Input: dimensioned drawing with shaded views. Units: mm. Origin: part minimum x, y, z. A direction names the side the tool comes from. Round coordinates to 2 decimals unless told otherwise and drop trailing zeros. Loops run counter-clockwise (first coordinate to the right, second up) from the corner with the lowest first, then second, coordinate; pieces in that order, holes last. Notation, with made-up numbers: (58.5, 38) -> (89.5, 38) arc R23 cw to (89.5, 76) -> close; hole circle Ø8 at (60, 79.25). An arc over 180 degrees is marked (long way). Answer as a JSON object with one key per item and string values.
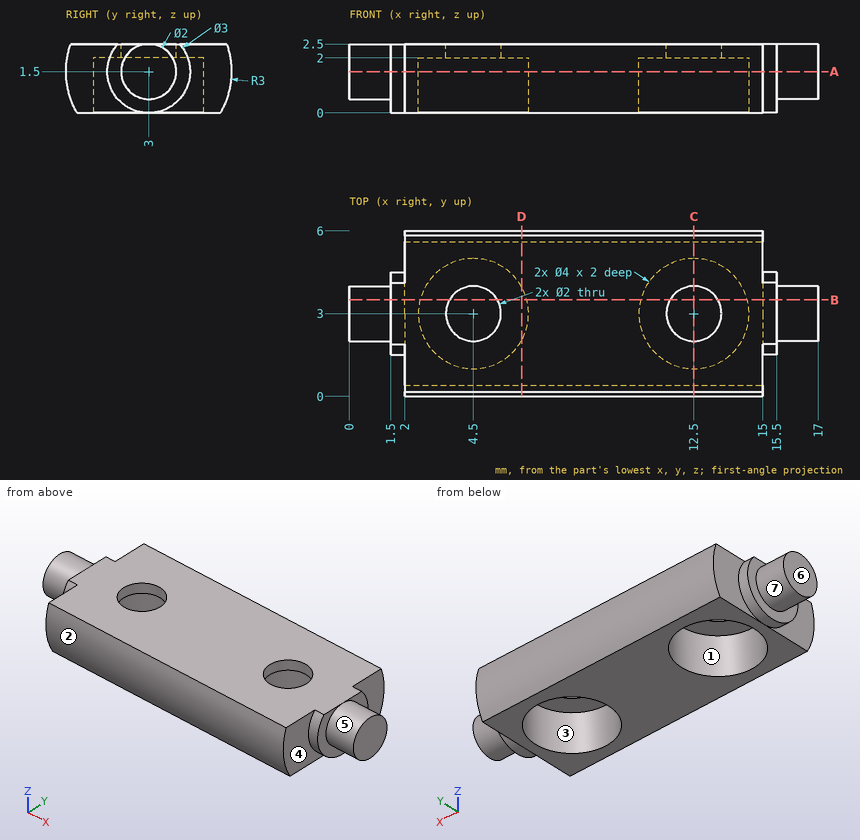
1) Reachability of the marked faces 5, 6 and 7 from +Z, -Z, +X, -X, +Y, -Y: full face, straight path, thin tool, end or side. Return the list, or none.
Output:
{"face 5": "+X", "face 6": "+Z, -Z, -X, +Y, -Y", "face 7": "-X"}
2) Section B-B, the plane y = 3.5. Count the separate pieces of the cut face and the enclosed holes in it, plus the area to 3 significant figures.
Output:
{"separate pieces": "3", "enclosed holes": "0", "area": "22.9 mm^2"}
3) Ray query, probe 1 along X at (y, z) = (3, 0.8); probe 2 along X at (y, z) = (1.5, 0.35); probe 3 along Y at (x, z) = (12.5, 1.4). Return the intervals inside material, ascending.
Output:
{"probe 1": "x = 0 to 2.5, 6.5 to 10.5, 14.5 to 17", "probe 2": "x = 2 to 3.18, 5.82 to 11.18, 13.82 to 15", "probe 3": "y = 0 to 1, 5 to 6"}
4) Contact query for flat-ended pins moving along their axis: P1, Ø1.5, axis at x = 15, z = 2, coming from the +Y side; P2, Ø2, axis at x = 13, y = 3.5, coming from the -Z side; P3, Ø0.8, axis at y = 5, z = 1.5, coming from the -X side. Output: stop coordinate, or through.
Output:
{"P1": "stops at y = 6", "P2": "stops at z = 2", "P3": "stops at x = 2"}
5) Section C-C, the plane x = 12.5. Output: boundary loops of the cut face in (y, z).
Output:
{"outline": "(0.17, 2.5) arc R3 ccw to (0.4, 0) -> (1, 0) -> (1, 2) -> (2, 2) -> (2, 2.5) -> close; (4, 2) -> (5, 2) -> (5, 0) -> (5.6, 0) arc R3 ccw to (5.83, 2.5) -> (4, 2.5) -> close"}
6) Section D-D, the plane x = 6.25. Output: boundary loops of the cut face in (y, z), plus the area to 3 significant figures.
Output:
{"outline": "(0.17, 2.5) arc R3 ccw to (0.4, 0) -> (2.03, 0) -> (2.03, 2) -> (3.97, 2) -> (3.97, 0) -> (5.6, 0) arc R3 ccw to (5.83, 2.5) -> close", "area": "10.6 mm^2"}
7) Draft query along X for the marked faces 1, 2, 3 and 4. Return one class per face: +X half, -X half, draft (parallel to the pull), parting line (faces both ways), or undercut.
Output:
{"face 1": "undercut", "face 2": "draft", "face 3": "undercut", "face 4": "+X half"}
8) Section A-A, the plane z = 1.5. Output: boundary loops of the cut face in (x, y), plus the area to 3 significant figures.
Output:
{"outline": "(0, 2) -> (1.5, 2) -> (1.5, 1.5) -> (2, 1.5) -> (2, 0) -> (15, 0) -> (15, 1.5) -> (15.5, 1.5) -> (15.5, 2) -> (17, 2) -> (17, 4) -> (15.5, 4) -> (15.5, 4.5) -> (15, 4.5) -> (15, 6) -> (2, 6) -> (2, 4.5) -> (1.5, 4.5) -> (1.5, 4) -> (0, 4) -> close; hole circle Ø4 at (4.5, 3); hole circle Ø4 at (12.5, 3)", "area": "61.9 mm^2"}
